from build123d import *

# Parameters (mm, degrees)
F_4_5_4_5_DIAMETER_HOLE1_D           = 4.5
F_4_5_4_5_DIAMETER_HOLE1_ON_FACE_2_D = 4.5
F_4_5_4_5_DIAMETER_HOLE2_D           = 4.5
F_4_5_4_5_DIAMETER_HOLE2_DEPTH       = 18
F_4_5_4_5_DIAMETER_HOLE2_TIP         = 1.351936393
CIRPATTERN1_COUNT                    = 4


with BuildPart() as part:
    # Esbo_o1 → Revolu_o1 (revolve)
    with BuildSketch(Plane.XY):
        Polygon((3, -9), (16, -9), (16, 5), (9, 5), (9, -5), (3, -5), align=None)
    revolve(axis=Axis((0, -9, 0), (0, 1, 0)))

    # 4.5 _4.5_ Diameter Hole1 (through all)
    with Locations(Plane(origin=(16, 0, 0), x_dir=(0, 0, 1), z_dir=(1, 0, 0))):
        with Locations((0, 0)):
            Hole(F_4_5_4_5_DIAMETER_HOLE1_D / 2)

    # 4.5 _4.5_ Diameter Hole1 on face 2 (through all)
    with Locations(Plane(origin=(0, 0, 0), x_dir=(0, 0, 1), z_dir=(1, 0, 0))):
        with Locations((0, 0)):
            Hole(F_4_5_4_5_DIAMETER_HOLE1_ON_FACE_2_D / 2)

    # 4.5 _4.5_ Diameter Hole2
    with Locations(Plane(origin=(-13.856406461, 0, -8), x_dir=(0, -1, 0), z_dir=(-0.866025404, 0, -0.5))):
        with Locations((0, 0)):
            Hole(F_4_5_4_5_DIAMETER_HOLE2_D / 2, depth=F_4_5_4_5_DIAMETER_HOLE2_DEPTH)
            with Locations((0, 0, -(F_4_5_4_5_DIAMETER_HOLE2_DEPTH + F_4_5_4_5_DIAMETER_HOLE2_TIP / 2))):  # 118° drill point
                Cone(0, F_4_5_4_5_DIAMETER_HOLE2_D / 2, F_4_5_4_5_DIAMETER_HOLE2_TIP, mode=Mode.SUBTRACT)

    # Sketch1 → M3x0.5 Tapped Hole1 (revolve, cut)
    with BuildSketch(Plane(origin=(-5.282728272, 5, -11.328847338), x_dir=(0, 0, 1), z_dir=(1, 0, 0))):
        Polygon((0, 0), (0, 12.751075774), (1.25, 12), (1.25, 0), align=None)
    m3x0_5_tapped_hole1 = revolve(axis=Axis((-5.282728272, 11.35, -11.328847338), (0, -1, 0)), mode=Mode.SUBTRACT)

    # CirPattern1: M3x0.5 Tapped Hole1 ×4 about axis
    cirpattern1_axis = Axis((0, 0, 0), (0, 1, 0))
    for i in range(1, CIRPATTERN1_COUNT):
        add(m3x0_5_tapped_hole1.rotate(cirpattern1_axis, i * 360 / CIRPATTERN1_COUNT), mode=Mode.SUBTRACT)


solid = part.part
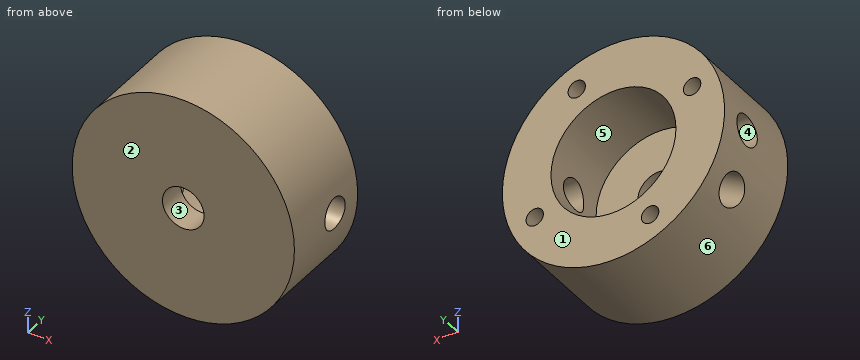
Work out the finished part from the listing and answer in its coordinate system (mm). Face numbers are marked on the shaded views. A direction names the side the tool comes from. Coordinates: 2 decimals unless noted, no trailing zeros. Write each loop counter-clockwise with the first axis right and the second up, starting at its lowest first coordinate (ties: lowest second). Pieces come first, ordered by that corner, then holes. Notation, with made-up numbers: M 13.5,-8.75 L 24.5,-8.75 A33 ccw 24.5,27.25 Z; hole C 44.5,-14 d6. An arc over 180 degrees is marked long. Use one line per item in the form item = value. Start each with the question number.
1. Straight lines are drawn through the part: probe 1 along Z at (x, y) = (5.5, -1); probe 2 along Z at (x, y) = (-5, 1.5); probe 3 along Y at (x, z) = (-10, 0). For each, find the intervals that lie inside material, in ascending order. Write a range as from..to.
2. The mould has two halves that part along Y. Classify the marked faces 1, 2, 3 and 4: released by +Y, released by -Y, zero draft, split by the parting line, or undercut.
3. The part is cut by section D-D (x = 14). Give the vertices of the cut face in (y, z), plus the area to 3 significant figures.
4. Each of these flat-tipped pins is pushed along its axis until it touches: P1, Ø1.5, axis at x = -1.5, y = -1.5, coming from the +Z side; P2, Ø4, axis at x = 5, y = -3, coming from the -Z side; P3, Ø16, axis at x = 0, z = 0, coming from the +Y side. Where does it stop, or does it pass through?
5. The part is cut by section B-B (x = 0). Give the vertices of the cut face in (y, z).
6. A tool of negligible diameter and unlimited length cuts with its end or side. For the marked faces 5 and 6, from which of +Z, -Z, +X, -X, +Y, -Y can it reach the whole face along a straight path? Write none if from no direction.
7. The part is cut by section C-C (z = 0). Give the vertices of the cut face in (x, y), plus the area to 3 significant figures.
8. The part is cut by section A-A (y = 0.75). Give the vertices of the cut face in (x, z), plus the area to 3 significant figures.
Evaluation:
q1.probe_1 = -15.02..-7.12, 7.12..10.1, 12.56..15.02
q1.probe_2 = -15.2..-12.55, -10.11..-7.48, 7.48..15.2
q1.probe_3 = -9..-2.25, 2.25..5
q2.face_1 = released by +Y
q2.face_2 = released by -Y
q2.face_3 = zero draft
q2.face_4 = undercut
q3.outline = M -9,-7.75 L 5,-7.75 L 5,7.75 L -9,7.75 Z; hole C 0,0 d4.5
q3.area = 201 mm^2
q4.P1 = 15.98
q4.P2 = -15.72
q4.P3 = -5
q5.outline = M -9,-16 L 5,-16 L 5,-9 L -5,-9 L -5,-3 L -9,-3 Z; M -9,3 L -5,3 L -5,9 L 5,9 L 5,16 L -9,16 Z
q6.face_5 = +Y
q6.face_6 = +Y, -Y
q7.outline = M -16,-9 L -3,-9 L -3,-5 L -9,-5 L -9,-2.25 L -16,-2.25 Z; M -16,2.25 L -9,2.25 L -9,5 L -16,5 Z; M 3,-9 L 16,-9 L 16,-2.25 L 9,-2.25 L 9,-5 L 3,-5 Z; M 9,2.25 L 16,2.25 L 16,5 L 9,5 Z
q7.area = 181 mm^2
q8.outline = M -15.86,-2.12 A16 ccw -14.79,-6.09 L -8.64,-2.54 A9 cw -8.75,-2.12 Z; M -15.86,2.12 L -8.75,2.12 A9 cw 8.75,2.12 L 15.86,2.12 A16 ccw Z; M -12.67,-9.77 A16 ccw 15.86,-2.12 L 8.75,-2.12 A9 cw -6.51,-6.21 Z; hole C -11.33,5.28 d2.5; hole C -5.28,-11.33 d2.5; hole C 5.28,11.33 d2.5; hole C 11.33,-5.28 d2.5
q8.area = 441 mm^2
